```python
from build123d import *


with BuildPart() as f2:
    # F2: sweep along a path in F0
    with BuildLine(Plane.XY) as f2_path:
        Line((0, 0), (140, 0))
        ThreePointArc((140, 0), (160, 20), (140, 40))
        Line((140, 40), (125, 40))
    # F1 (on Right) → F2 (sweep)
    with BuildSketch(Plane.YZ):
        Polygon((0, 15), (0, 0), (10, 0), (10, 3), (3, 3), (3, 15), align=None)
    sweep(path=f2_path.line)


solid = f2.part
```
For this review, take the finished solid that the model builds, in its own axes (mm). A direction names the side the tool comes from. Round coordinates to 2 decimals unless told otherwise and drop trailing zeros. Write each loop counter-clockwise with the first axis right and the second up, starting at its lowest first coordinate (ties: lowest second). Pieces come first, ordered by that corner, then holes. Notation, with made-up numbers: (64, 2) - (105, 2) arc R33 ccw to (105, 32) - close; hole circle Ø1 at (-33, 32.5). An arc over 180 degrees is marked (long way). Answer as a JSON object with one key per item and string values.
1. We need section B-B on x = 29. Give the boundary of the cut face in (y, z).
Response values:
{"outline": "(0, 0) - (10, 0) - (10, 3) - (3, 3) - (3, 15) - (0, 15) - close"}
2. Draft analysis for pull direction Y (two halves, no side actions). For faces 1 (the face through (132, 37, 9)), 2 (the face through (125, 37.2, 5.9)), 3 (the face through (160, 20, 7)), 4 (the face through (157, 20, 9)), state which applies: +Y half, -Y half, draft (parallel to the pull), parting line (faces both ways), or undercut.
Response values:
{"face 1": "undercut", "face 2": "draft", "face 3": "parting line", "face 4": "undercut"}
3. We need section C-C on y = 20. Give the boundary of the cut face in (x, z).
Response values:
{"outline": "(150, 0) - (160, 0) - (160, 15) - (157, 15) - (157, 3) - (150, 3) - close"}
4. To check wall thickness, follow line 1 along Y through (x, z) = (126.5, 9.75); line 2 along Y through (x, z) = (99, 10). State the ranges of each line that lie inside material, in increasing order.
Response values:
{"line 1": "y = 0 to 3, 37 to 40", "line 2": "y = 0 to 3"}
5. Tool access review of faces 5 (the face through (96, 9, 3)), 6 (the face through (132, 30, 1)), 7 (the face through (132, 40, 8)): name each direction out of +Z, -Z, +X, -X, +Y, -Y from which nothing blocks a thin tool from reaching the whole face with its end or side.
Response values:
{"face 5": "+Z, -X", "face 6": "+Z, -Z, -X", "face 7": "+Z, -Z, +X, -X, +Y"}
6. We need section A-A on z = 10.5. Give the boundary of the cut face in (x, y), then the cut area to 3 significant figures.
Response values:
{"outline": "(0, 0) - (140, 0) arc R20 ccw to (140, 40) - (125, 40) - (125, 37) - (140, 37) arc R17 cw to (140, 3) - (0, 3) - close", "area": "639 mm2"}
7. For pin 1 Ø8 at (y, z) = (33.5, 7) entering from -X; pin 2 Ø2.5 at (x, z) = (71, 1) entering from +Y; pin 3 Ø3 at (x, z) = (109.5, 12.5) entering from +Y, all flat-tipped, find the tip position at first contact; note any pin that passes through.
Response values:
{"pin 1": "stops at x = 125", "pin 2": "stops at y = 10", "pin 3": "stops at y = 3"}
